Here's how the part is built. I have some questions about the finished solid (model axes, mm). A direction names the side the tool comes from. Coordinates: 2 decimals unless noted, no trailing zeros. Loops run counter-clockwise (first coordinate to the right, second up) from the corner with the lowest first, then second, coordinate; pieces in that order, holes last. Notation, with made-up numbers: (49.25, 57) -> (100.25, 57) arc R25 cw to (100.25, 85) -> close; hole circle Ø9 at (20.5, 70). An arc over 180 degrees is marked (long way). Use CSV: the item, a comma, the result in double quotes. Start each with the question number.
Autodesk Inventor part; units mm, degrees
ref_plane "YZ Plane" through (0, 0, 0) normal (1, 0, 0) x (0, 1, 0)
ref_plane "XZ Plane" through (0, 0, 0) normal (0, 1, 0) x (-1, 0, 0)
ref_plane "XY Plane" through (0, 0, 0) normal (0, 0, 1) x (1, 0, 0)
sketch "Sketch1" plane through (0, 0, 0) normal (0, 1, 0) x (-1, 0, 0)
  circle A0 centre (0, 0) radius 90
  line L0 (55, -71.239) -> (55, 71.239)
  dimension "d0" = 180
  dimension "d1" = 55
extrude "Extrusion1" add sketch "Sketch1" along normal blind 3 contours L0 A0 picked at (6.6667, 0)
sketch "Sketch2" plane through (0, 3, 0) normal (0, 1, 0) x (1, 0, 0)
  arc A0 (-55, -71.239) -> (-55, 71.239) centre (0, 0) ccw
  line L0 (-52, 73.4575) -> (-52, -73.4575)
  line L1 (-55, 71.239) -> (-55, -71.239)
  dimension "d4" = 3
extrude "Extrusion2" cut sketch "Sketch2" against normal blind 3 contours L1 A0 L0
sketch "Sketch3" plane through (0, 3, 0) normal (0, 1, 0) x (1, 0, 0)
  line L0 (-52, 73.4575) -> (-52, -73.4575)
  arc A0 (-52, -73.4575) -> (-52, 73.4575) centre (0, 0) ccw
  line L1 (-32, -62.2575) -> (-32, 62.2575)
  arc A1 (-32, -62.2575) -> (-32, 62.2575) centre (0, 0) ccw
  dimension "d7" = 20
extrude "Extrusion3" cut sketch "Sketch3" against normal blind 3 contours L1 A1
sketch "Sketch4" plane through (0, 3, 0) normal (0, 1, 0) x (1, 0, 0)
  arc A0 (-32, -62.2575) -> (-32, 62.2575) centre (0, 0) ccw
  line L0 (51, -47.9479) -> (76.1643, -47.9479)
  line L1 (76.1643, -47.9479) -> (76.1643, 47.9479)
  line L2 (76.1643, 47.9479) -> (51, 47.9479)
  line L3 (51, 47.9479) -> (51, -47.9479)
  line L4 (-52, 73.4575) -> (-52, -73.4575)
  arc A1 (-52, -73.4575) -> (-52, 73.4575) centre (0, 0) ccw
  dimension "d10" = 103
extrude "Extrusion4" add sketch "Sketch4" against normal blind 3 contours L3 A0
sketch "Sketch5" plane through (0, 3, 0) normal (0, 1, 0) x (1, 0, 0)
  line L0 (48, -19) -> (64, -19)
  line L1 (64, -19) -> (64, 19)
  line L2 (64, 19) -> (48, 19)
  line L3 (48, 19) -> (48, -19)
  line L4 (-52, 73.4575) -> (-52, -73.4575)
  point P0 (0, 0)
  point P1 (64, 0)
  dimension "d13" = 16
  dimension "d14" = 38
  dimension "d15" = 100
extrude "Extrusion5" cut sketch "Sketch5" against normal blind 3
sketch "Sketch6" plane through (0, 3, 0) normal (0, 1, 0) x (1, 0, 0)
  line L0 (64, -24) -> (43, -24)
  line L1 (43, -24) -> (43, 24)
  line L2 (43, 24) -> (64, 24)
  line L3 (64, 24) -> (64, -24)
  line L4 (-52, 73.4575) -> (-52, -73.4575)
  arc A0 (-52, -73.4575) -> (-52, 73.4575) centre (0, 0) ccw
  line L5 (51, 19) -> (64, 19)
  line L6 (64, 19) -> (64, -19)
  line L7 (64, -19) -> (51, -19)
  line L8 (51, -19) -> (51, -47.9479)
  arc A1 (-32, -62.2575) -> (51, -47.9479) centre (0, 0) ccw
  line L9 (-32, -62.2575) -> (-32, 62.2575)
  arc A2 (51, 47.9479) -> (-32, 62.2575) centre (0, 0) ccw
  line L10 (51, 47.9479) -> (51, 19)
  line L11 (64, -19) -> (48, -19)
  line L12 (48, -19) -> (48, 19)
  line L13 (48, 19) -> (64, 19)
  line L14 (64, 19) -> (64, -19)
  line L15 (51, 19) -> (64, 19)
  line L16 (64, 19) -> (64, -19)
  dimension "d18" = 5
  dimension "d19" = 5
  dimension "d20" = 8
  dimension "d21" = 16
extrude "Extrusion6" add sketch "Sketch6" against normal blind 3 contours L0 L8 L7 L3 | L0 L1 L2 L10 L13 L12 L11 L8 | L5 L10 L2 L3
sketch "Sketch7" plane through (0, 3, 0) normal (0, 1, 0) x (1, 0, 0)
  line L0 (43, 24) -> (51, 24)
  line L1 (48, 24) -> (51, 24)
  line L2 (51, 24) -> (51, 60)
  line L3 (51, 60) -> (48, 60)
  line L4 (48, 60) -> (48, 24)
  line L5 (51, 47.9479) -> (51, 24)
  line L6 (48, 60) -> (36.0555, 60)
  line L7 (36.0555, 60) -> (36.0555, 50.951)
  line L8 (36.0555, 50.951) -> (48, 50.951)
  line L9 (48, 50.951) -> (48, 60)
  arc A0 (51, 47.9479) -> (-32, 62.2575) centre (0, 0) ccw
  dimension "d24" = 3
  dimension "d25" = 36
extrude "Extrusion7" cut sketch "Sketch7" against normal blind 3
sketch "Sketch8" plane through (0, 3, 0) normal (0, 1, 0) x (1, 0, 0)
  line L0 (51, 60) -> (51, 24)
  line L1 (51, 47) -> (48, 47)
  line L2 (48, 47) -> (48, 37)
  line L3 (48, 37) -> (51, 37)
  line L4 (51, 37) -> (51, 47)
  line L5 (36.0555, 60) -> (51, 60)
  point P0 (0, 0)
  dimension "d28" = 3
  dimension "d29" = 10
  dimension "d30" = 13
extrude "Extrusion8" add sketch "Sketch8" against normal blind 3
mirror "Mirror1" about plane through (0, 0, 0) normal (0, 0, 1) of "Extrusion8", "Extrusion7"
equation "\"d19\" = d18"
properties part number "suport plate"
1) Which directions (+Z, -Z, +X, -X, +Y, -Y) give clear straight access to the entire face, cutting with the end or side of a thin tool? Please do faces 1 (the face through (52, 0, 21)), 2 (the face through (1.823, 1.521, 69.976)).
2) Thinking about a two-plate mould opening in Z: for faces 3 (the face through (2.818, 1.521, -69.943)), 4 (the face through (52, 3, 21)), 5 (the face through (89.958, 1.479, -2.755)), which applies, pulls with the +Z half, pulls with the -Z half, needs draft (parallel to the pull), parting line crosses it, or undercut?
3) I want a section at A-A, the plane x = 0. Please give me the cut outline in (y, z).
4) I want a section at D-D, the plane z = -50. Please give me the cut outline in (x, y), plus the area to 3 significant figures.
5) For P1, Ø0.9, axis at x = 60, y = 1.5, coming from the +Z side; P2, Ø1.5, axis at x = -4.5, y = 2.5, coming from the +Z side; P3, Ø1.5, axis at x = 47, y = 2, coming from the +Z side, each with a flat end and sliding along its axis, tell me the tip position at first contact or that it passes through.
6) Please list where these lines run through material, in increasing order: L1, parallel to X at y = 2.35, z = -2.5; L2, parallel to Z at x = 8.5, y = 2.05; L3, parallel to X at y = 1.8, z = 59.5. Write a range as [from, to].
7) I want a section at C-C, the plane y = 1.4. Please give me the cut outline in (x, z), plus the area to 3 significant figures.
8) I want a section at B-B, the plane z = 0. Please give me the cut outline in (x, y).
Return value:
1,face 1,"+Z, -Z, +X, -X, -Y"
1,face 2,"+Y, -Y"
2,face 3,"undercut"
2,face 4,"needs draft"
2,face 5,"parting line crosses it"
3,outline,"(0, -90) -> (3, -90) -> (3, -70) -> (0, -70) -> close; (0, 70) -> (3, 70) -> (3, 90) -> (0, 90) -> close"
4,outline,"(-52, 0) -> (-32, 0) -> (-32, 3) -> (-52, 3) -> close; (51, 0) -> (74.83, 0) -> (74.83, 3) -> (51, 3) -> close"
4,area,"131 mm²"
5,P1,"stops at z = 67.48"
5,P2,"stops at z = 89.92"
5,P3,"stops at z = 77.21"
6,L1,"x = [-52, -32], [43, 48], [64, 89.97]"
6,L2,"z = [-89.6, -69.48], [69.48, 89.6]"
6,L3,"x = [-52, -32], [51, 67.53]"
7,outline,"(-52, -73.46) arc R90 ccw (long way) to (-52, 73.46) -> close; hole (-32, -62.26) arc R70 ccw to (36.06, -60) -> (51, -60) -> (51, -47) -> (48, -47) -> (48, -37) -> (51, -37) -> (51, -24) -> (43, -24) -> (43, 24) -> (51, 24) -> (51, 37) -> (48, 37) -> (48, 47) -> (51, 47) -> (51, 60) -> (36.06, 60) arc R70 ccw to (-32, 62.26) -> close; hole (48, -19) -> (64, -19) -> (64, 19) -> (48, 19) -> close"
7,area,"10,400 mm²"
8,outline,"(-52, 0) -> (-32, 0) -> (-32, 3) -> (-52, 3) -> close; (43, 0) -> (48, 0) -> (48, 3) -> (43, 3) -> close; (64, 0) -> (90, 0) -> (90, 3) -> (64, 3) -> close"
